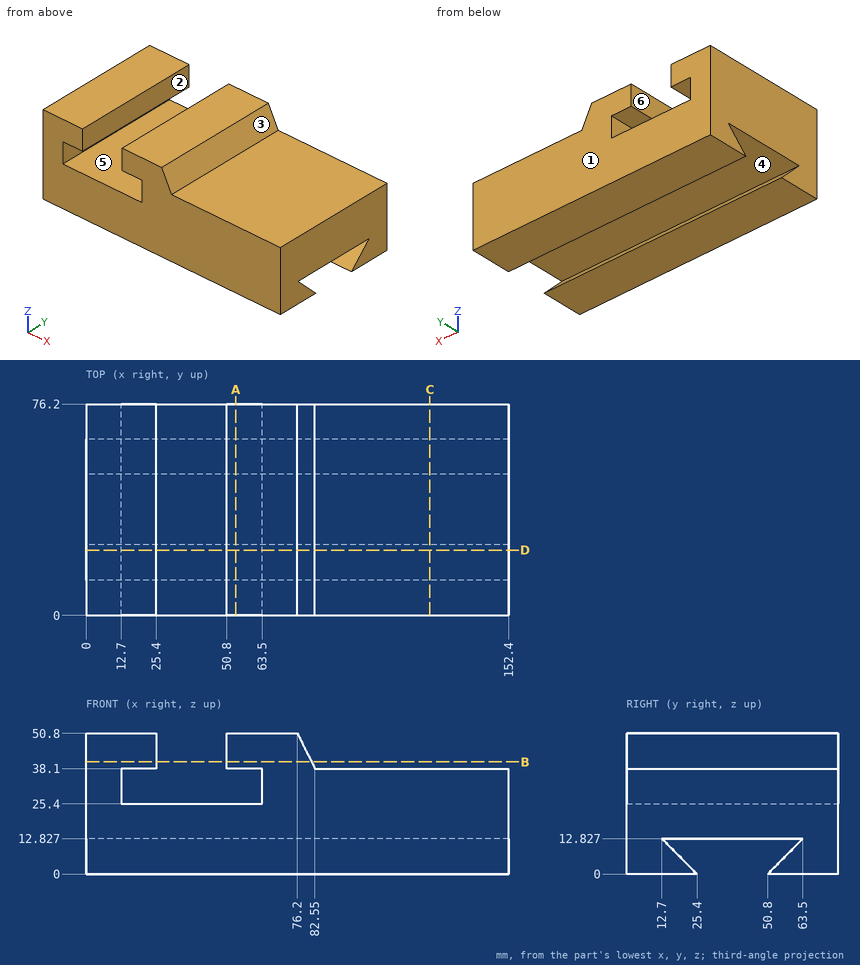
Can you work these out from the drawing? Everything is in mm from the part's minimum corner. A direction names the side the tool comes from. Round coordinates to 2 decimals unless told otherwise and drop trailing zeros. Write each loop counter-clockwise with the first axis right and the second up, starting at its lowest first coordinate (ties: lowest second). Pieces come first, ordered by that corner, then holes. Notation, with made-up numbers: (-9.5, 27.25) - (47.5, 27.25) arc R18 ccw to (47.5, 39.25) - close; hole circle Ø10 at (80.5, 13.25). An arc over 180 degrees is marked (long way). Put each result on its own line as item: value. Start each with the question number.
(1) I want a section at D-D, the plane y = 23.5. Please give me the cut outline in (x, z).
(2) I want a section at C-C, the plane x = 124. Please give me the cut outline in (y, z), plus the area to 3 significant figures.
(3) I want a section at B-B, the plane z = 40.5. Please give me the cut outline in (x, y).
(4) I need wall thicknesses on probe 1 along X at (y, z) = (68, 31.5); probe 2 along Z at (x, y) = (57.5, 39); probe 3 along Z at (x, y) = (24, 62). Which ranges of each line are inside material? Lowest first, please.
(5) Will these pins go through, and if not, where does the flat tip stop? pin 1 (1.5 mm diameter, centred on x = 39, y = 59, fed in from +Z); pin 2 (10 mm diameter, centred on y = 38.5, z = 46.5, fed in from +X); pin 3 (14 mm diameter, centred on x = 54, y = 42, fed in from -Z).
(6) For the marked faces 4, 5 and 6, which set-ups out of +Z, -Z, +X, -X, +Y, -Y let a thin tool reach every point of the face, with its end or its side?
(7) I want a section at A-A, the plane x = 54. Please give me the cut outline in (y, z), plus the area to 3 significant figures.
(8) Thinking about a two-plate mould opening in X: for the marked faces 1, 2 and 3, which applies, released by +X, released by -X, zero draft, split by the parting line, or undercut?
Here are the results:
1. outline: (0, 0) - (152.4, 0) - (152.4, 1.92) - (0, 1.92) - close; (0, 12.83) - (152.4, 12.83) - (152.4, 38.1) - (82.55, 38.1) - (76.2, 50.8) - (50.8, 50.8) - (50.8, 38.1) - (63.5, 38.1) - (63.5, 25.4) - (12.7, 25.4) - (12.7, 38.1) - (25.4, 38.1) - (25.4, 50.8) - (0, 50.8) - close
2. outline: (0, 0) - (25.4, 0) - (12.7, 12.83) - (63.5, 12.83) - (50.8, 0) - (76.2, 0) - (76.2, 38.1) - (0, 38.1) - close
2. area: 2,410 mm^2
3. outline: (0, 0) - (25.4, 0) - (25.4, 76.2) - (0, 76.2) - close; (50.8, 0) - (81.35, 0) - (81.35, 76.2) - (50.8, 76.2) - close
4. probe 1: x = 0 to 12.7, 63.5 to 152.4
4. probe 2: z = 12.83 to 25.4, 38.1 to 50.8
4. probe 3: z = 0 to 11.31, 12.83 to 25.4, 38.1 to 50.8
5. pin 1: stops at z = 25.4
5. pin 2: stops at x = 80.85
5. pin 3: stops at z = 12.83
6. face 4: +X, -X
6. face 5: +Y, -Y
6. face 6: +Z, +Y, -Y
7. outline: (0, 0) - (25.4, 0) - (12.7, 12.83) - (63.5, 12.83) - (50.8, 0) - (76.2, 0) - (76.2, 25.4) - (0, 25.4) - close; (0, 38.1) - (76.2, 38.1) - (76.2, 50.8) - (0, 50.8) - close
7. area: 2,410 mm^2
8. face 1: zero draft
8. face 2: undercut
8. face 3: released by +X
